from build123d import *

# Parameters (mm, degrees)
BOSS_EXTRUDE6_START       = -141.338468014
BOSS_EXTRUDE6_DEPTH       = 27.296026611
BOSS_EXTRUDE6_START_2     = -101.470072675
BOSS_EXTRUDE6_2_OUTLINE_W = 72
BOSS_EXTRUDE6_2_OUTLINE_H = 103
BOSS_EXTRUDE6_2_DEPTH     = 23.568848061
BOSS_EXTRUDE6_START_3     = -127.947953139
BOSS_EXTRUDE6_3_OUTLINE_W = 72
BOSS_EXTRUDE6_3_OUTLINE_H = 103
BOSS_EXTRUDE6_3_DEPTH     = 23.567768302
SKETCH1_R                 = 2.5
BOSS_EXTRUDE8_DEPTH       = 3


with BuildPart() as part:
    # Boss-Extrude6: read off the stored shape, not the designer's step
    # Boss-Extrude6 outline → Boss-Extrude6 (new body)
    with BuildSketch(Plane.YZ.offset(BOSS_EXTRUDE6_START)):
        Polygon((86.01064189, 134.693213905), (17.476837079, 134.693213905), (17.476837075, 37.689278418), (86.008364377, 37.690000992), align=None)
    extrude(amount=BOSS_EXTRUDE6_DEPTH)

    # Boss-Extrude6 2 outline → Boss-Extrude6 2 (cut)
    with BuildSketch(Plane(origin=(0, 0, 0), x_dir=(1.5283083166138014e-05, 0.9999999998758877, 3.827802984502311e-06), z_dir=(0.9700373872996308, -1.5755148579155195e-05, 0.24295568936059395)).offset(BOSS_EXTRUDE6_START_2)):
        with Locations((52, 114.5)):
            Rectangle(BOSS_EXTRUDE6_2_OUTLINE_W, BOSS_EXTRUDE6_2_OUTLINE_H)
    extrude(amount=BOSS_EXTRUDE6_2_DEPTH, mode=Mode.SUBTRACT)

    # Boss-Extrude6 3 outline → Boss-Extrude6 3 (cut)
    with BuildSketch(Plane(origin=(0, 0, 0), x_dir=(1.5283083166138014e-05, 0.9999999998758877, 3.827802984502311e-06), z_dir=(0.9700373872996308, -1.5755148579155195e-05, 0.24295568936059395)).offset(BOSS_EXTRUDE6_START_3)):
        with Locations((52, 114.5)):
            Rectangle(BOSS_EXTRUDE6_3_OUTLINE_W, BOSS_EXTRUDE6_3_OUTLINE_H)
    extrude(amount=BOSS_EXTRUDE6_3_DEPTH, mode=Mode.SUBTRACT)

    # Sketch1 → Boss-Extrude8 (add)
    with BuildSketch(Plane.XZ.offset(-17.476837075)):
        Polygon((-138.338991718, 134.693148321), (-130.338991718, 134.693148321), (-106.043946484, 37.689278418), (-114.043946484, 37.689278418), (-117.043946484, 37.689278418), (-141.338991718, 134.693148321), align=None)
        with Locations(Location((-132.458903411, 126.693148321, 0), (0, 0, 270))):
            Circle(SKETCH1_R, mode=Mode.SUBTRACT)
        with Locations(Location((-112.171128445, 45.689278418, 0), (0, 0, 270))):
            Circle(SKETCH1_R, mode=Mode.SUBTRACT)
    extrude(amount=-BOSS_EXTRUDE8_DEPTH)


solid = part.part
Read the model definition and answer for the solid it produces. Units are mm, in the model's axes. A direction names the side the tool comes from. Round coordinates to 2 decimals unless told otherwise and drop trailing zeros. Write each loop counter-clockwise with the first axis right and the second up, starting at its lowest first coordinate (ties: lowest second). Pieces come first, ordered by that corner, then holes.
Q1. The mould has two halves that part along Z. Classify faces 3 (the face through (-118.36, 18.96, 86.87)), 4 (the face through (-112, 19, 37.689)), 5 (the face through (-130.35, 18.96, 125.35)): released by +Z, released by -Z, zero draft, split by the parting line, or undercut.
Values:
face 3: released by +Z
face 4: released by -Z
face 5: undercut
Q2. Find section A-A on x = -133.5. Determine the outline of the cut face in (y, z), and give its area (3 significant figures).
Values:
outline: (17.48, 103.39) - (86.01, 103.4) - (86.01, 115.38) - (20.48, 115.37) - (20.48, 124.42) - (17.48, 124.42) - close; (17.48, 128.97) - (20.48, 128.97) - (20.48, 134.69) - (17.48, 134.69) - close
area: 865 mm2
Q3. Flat-ended cylindrical pins translate along their axes: P1, Ø1.5, axis at y = 70.5, z = 103, coming from the +X side; P2, Ø1.5, axis at y = 58.5, z = 124.5, coming from the -X side; P3, Ø1.5, axis at y = 51, z = 56.5, coming from the +X side. Find the tip coordinate at first contact, or state that the pin passes through.
Values:
P1: stops at x = -130.21
P2: stops at x = -138.97
P3: stops at x = -118.57
Q4. A tool of negligible diameter and unlimited length cuts with its end or side. For faces 1 (the face through (-134, 19, 134.693)), 2 (the face through (-122, 20.477, 86)), from which of +Z, -Z, +X, -X, +Y, -Y can it reach the whole face along a straight path? Write none if from no direction.
Values:
face 1: +Z, +X, -X, +Y, -Y
face 2: +Z, +X, +Y
Q5. Straight lines are drawn through the part: line 1 (Y direction, x = -115.5, z = 58); line 2 (X direction, y = 81.5, z = 45.5); line 3 (X direction, y = 59, z = 90). For each, find the intervals that lie inside material, in ascending order.
Values:
line 1: y = 17.48 to 20.48
line 2: x = -119 to -116
line 3: x = -130.14 to -127.14
Q6. Find section C-C on z = 120. Determine the outline of the cut face in (x, y).
Values:
outline: (-137.66, 17.48) - (-126.66, 17.48) - (-126.66, 20.48) - (-134.66, 20.48) - (-134.66, 86.01) - (-137.66, 86.01) - close
